Drawing for the job (mm, zero at the part's lowest x, y, z). A direction names the side the tool comes from. Coordinates: 2 decimals unless noted, no trailing zeros. Order: outer loops, then holes, each group sorted by start corner. A loop starts at its lowest first (then second) coordinate and runs counter-clockwise, first axis right, second up. Notation, with made-up numbers: (7.25, 79) -> (59.25, 79) arc R30 cw to (59.25, 115) -> close; hole circle Ø5 at (-5, -12). An arc over 180 degrees is marked (long way). Write each question's results on one line, items separated by ' | '.
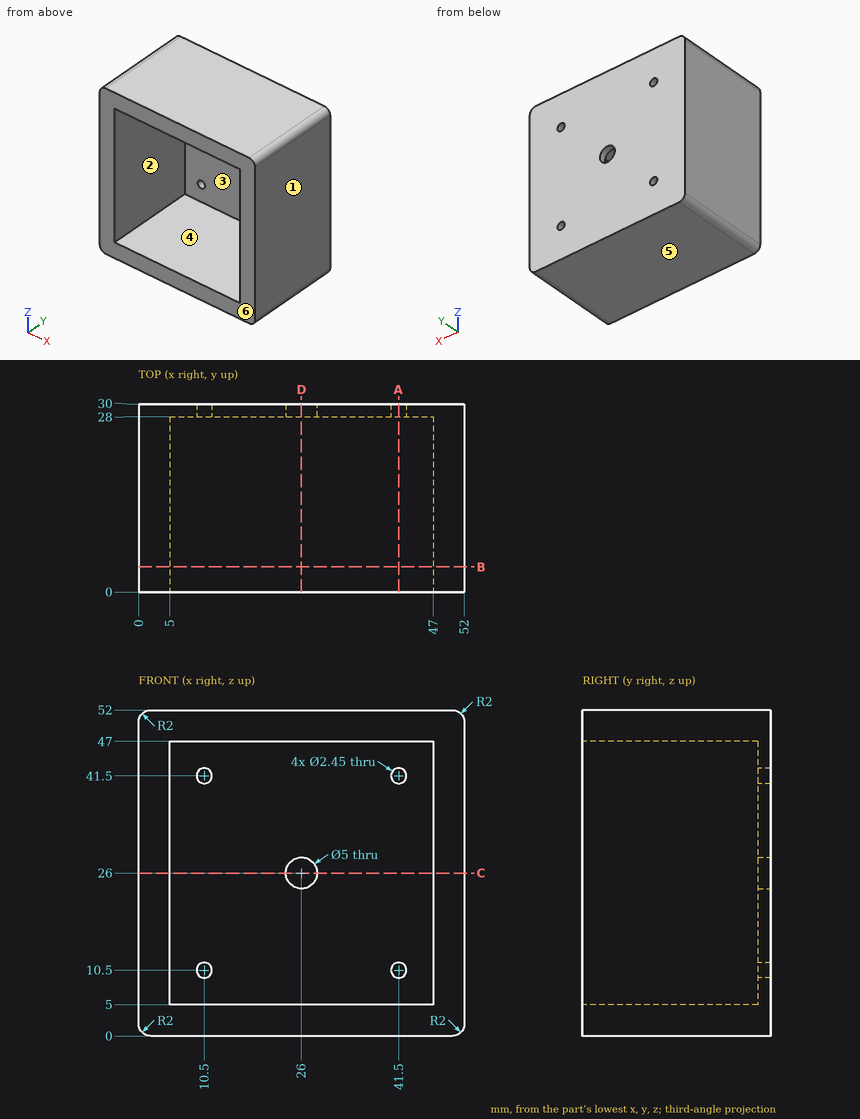
Item 1: Slice it at B-B, the plane y = 4. List the corners of the cut face in (x, z).
Answer:
outline: (0, 2) arc R2 ccw to (2, 0) -> (50, 0) arc R2 ccw to (52, 2) -> (52, 50) arc R2 ccw to (50, 52) -> (2, 52) arc R2 ccw to (0, 50) -> close; hole (5, 5) -> (47, 5) -> (47, 47) -> (5, 47) -> close
Item 2: Pull direction Z, two halves, no side cores. Call the marked faces 3, 4, 5 and 6: released by +Z, released by -Z, zero draft, split by the parting line, or undercut.
Answer:
face 3: undercut | face 4: undercut | face 5: released by -Z | face 6: zero draft
Item 3: Pin check, flat tip, straight feed: pin 1 (4 mm diameter, centred on x = 10.5, z = 41.5, fed in from -Y). Stop position of the tip, or through.
Answer:
pin 1: stops at y = 28
Item 4: Slice it at C-C, the plane z = 26. List the corners of the cut face in (x, y), and give its area (3 significant figures).
Answer:
outline: (0, 0) -> (5, 0) -> (5, 28) -> (23.5, 28) -> (23.5, 30) -> (0, 30) -> close; (28.5, 28) -> (47, 28) -> (47, 0) -> (52, 0) -> (52, 30) -> (28.5, 30) -> close | area: 374 mm^2
Item 5: Slice it at A-A, the plane x = 41.5. List the corners of the cut face in (y, z) (3 decimals), and give its area (3 significant figures).
Answer:
outline: (0, 0) -> (30, 0) -> (30, 9.275) -> (28, 9.275) -> (28, 5) -> (0, 5) -> close; (0, 47) -> (28, 47) -> (28, 42.725) -> (30, 42.725) -> (30, 52) -> (0, 52) -> close; (28, 11.725) -> (30, 11.725) -> (30, 40.275) -> (28, 40.275) -> close | area: 374 mm^2
Item 6: Slice it at D-D, the plane x = 26. List the corners of the cut face in (y, z).
Answer:
outline: (0, 0) -> (30, 0) -> (30, 23.5) -> (28, 23.5) -> (28, 5) -> (0, 5) -> close; (0, 47) -> (28, 47) -> (28, 28.5) -> (30, 28.5) -> (30, 52) -> (0, 52) -> close
Item 7: Tool access for the marked faces 1 and 2: list every direction of +Z, -Z, +X, -X, +Y, -Y with a clear straight run to the whole face (end or side of a thin tool).
Answer:
face 1: +Z, -Z, +X, +Y, -Y | face 2: -Y
Item 8: Drill centre lines: line 1 (Z direction, x = 10.5, y = 28.55) (3 decimals); line 2 (X direction, y = 12.5, z = 25). Where is each one in solid material? Low to high. Write a range as from..to.
Answer:
line 1: z = 0..9.275, 11.725..40.275, 42.725..52 | line 2: x = 0..5, 47..52
